Geometry check sheet. Reference: drawing and pictorial views, mm from the part's lowest x, y, z. Give positions to 0.01 mm unless a question says otherwise; leave off trailing zeros. Order: outer loops, then holes, each group sorted by start corner. A loop starts at its lowest first (then second) coordinate and runs counter-clockwise, first axis right, second up. Notation, with made-up numbers: (23.25, 88) - (52.25, 88) arc R23 cw to (52.25, 111) - close; hole circle Ø2 at (35.25, 37). An arc over 180 degrees is marked (long way). Answer in a Markdown table with one row per item.
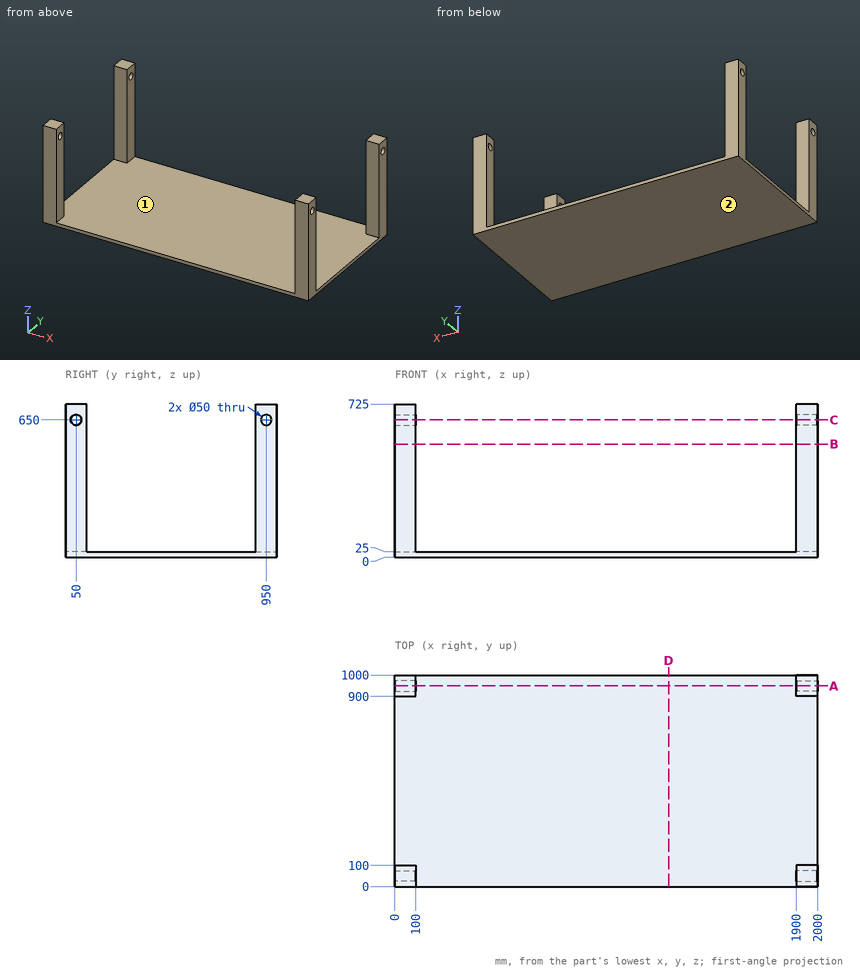
(1) Cross-section at C-C, the plane z = 650. Give the number of separate pieces and of enclosed holes in the cut face, then the cut area to 3 significant figures.
Geometry says:
| item | result |
|---|---|
| separate pieces | 8 |
| enclosed holes | 0 |
| area | 20,000 mm² |
(2) Thickness scan on L1, parallel to X at y = 958, z = 498.5; L2, parallel to Z at x = 48, y = 50; L3, parallel to Z at x = 385.5, y = 83. Record the ranges inside material, lowest first.
Geometry says:
| item | result |
|---|---|
| L1 | 0 to 100, 1900 to 2000 |
| L2 | 0 to 625, 675 to 725 |
| L3 | 0 to 25 |
(3) Cross-section at A-A, the plane y = 950. Record the cut outline in (x, z), then the cut area to 3 significant figures.
Geometry says:
| item | result |
|---|---|
| outline | (0, 0) - (2000, 0) - (2000, 625) - (1900, 625) - (1900, 25) - (100, 25) - (100, 625) - (0, 625) - close; (0, 675) - (100, 675) - (100, 725) - (0, 725) - close; (1900, 675) - (2000, 675) - (2000, 725) - (1900, 725) - close |
| area | 180,000 mm² |
(4) Cross-section at D-D, the plane x = 1296. Record the cut outline in (y, z).
Geometry says:
| item | result |
|---|---|
| outline | (0, 0) - (1000, 0) - (1000, 25) - (0, 25) - close |
(5) Gauge pin test, flat end, axial feed: P1, Ø6, axis at x = 1222, y = 312.5, coming from the +Z side. Record the tip position at first contact, or that the pin passes through.
Geometry says:
| item | result |
|---|---|
| P1 | z = 25 |
(6) Mould release check, pull along X, two halves, no side actions. Record for the marked faces 1 and 2: pulls with the +X half, pulls with the -X half, needs draft (parallel to the pull), parting line crosses it, or undercut.
Geometry says:
| item | result |
|---|---|
| face 1 | undercut |
| face 2 | needs draft |
(7) Cross-section at B-B, the plane z = 535. Record the cut outline in (x, y), then the cut area to 3 significant figures.
Geometry says:
| item | result |
|---|---|
| outline | (0, 0) - (100, 0) - (100, 100) - (0, 100) - close; (0, 900) - (100, 900) - (100, 1000) - (0, 1000) - close; (1900, 0) - (2000, 0) - (2000, 100) - (1900, 100) - close; (1900, 900) - (2000, 900) - (2000, 1000) - (1900, 1000) - close |
| area | 40,000 mm² |
